Could you check a few things on this model? Use its own coordinates, in mm. A direction names the side the tool comes from. Round coordinates to 2 decimals unless told otherwise and drop trailing zeros. Loops run counter-clockwise (first coordinate to the right, second up) from the corner with the lowest first, then second, coordinate; pieces in that order, holes last. Notation, with made-up numbers: M -37.75,88 L 3.25,88 A24 ccw 3.25,114 Z; hole C 19.5,-32.75 d5. An arc over 180 degrees is marked long. One line per item, written item: value. Start each with the question number.
Q1. Imagine slicing it at D-D (y = 6.25). Please give me the cut outline in (x, z), then the cut area to 3 significant figures.
Q2. Imagine slicing it at B-B (z = 28). Please give me the cut outline in (x, y).
Q3. Which directions (+Z, -Z, +X, -X, +Y, -Y) give clear straight access to the entire face, cutting with the end or side of a thin tool? Please do faces 1 (the face through (12, 7, 19)), 2 (the face through (5, 0.5, 40)), 3 (the face through (14.5, 8, 40)).
Q4. Imagine slicing it at C-C (x = -4.5). Please give me the cut outline in (y, z), then the cut area to 3 significant figures.
Q5. Imagine slicing it at A-A (y = 9). Please give me the cut outline in (x, z), then the cut area to 3 significant figures.
Q6. I'm going to push flat-ended pins straight in: pin 1 Ø6 at (x, y) = (10.5, 4.5) entering from +Z; pin 2 Ø0.6 at (x, z) = (13, 40) entering from +Y; pin 3 Ø6 at (x, y) = (-9.5, 5.5) entering from -Z; pin 4 Ø12 at (x, z) = (4, 30) entering from +Y. Where does each tip first touch, or does it pass through?
Q7. Thinking about a two-plate mould opening in X: for faces 4 (the face through (-15, 5, 20)), 5 (the face through (0, 3, 19)), 6 (the face through (12, 0.5, 40)), which applies, released by +X, released by -X, zero draft, split by the parting line, or undercut?
Q8. Please list where these lines run through material, in increasing order: line 1 along X through (y, z) = (4.75, 29); line 2 along Y through (x, z) = (-9.5, 6.5); line 3 along Z through (x, y) = (-8.25, 1.25).
from build123d import *

# Parameters (mm, degrees)
F1_DEPTH = 39
F2_W     = 0.5
F2_H     = 3
F2_W_2   = 5
F2_H_2   = 0.5
F2_W_3   = 3
F3_DEPTH = 2


with BuildPart() as f1:
    # F0 (on Top) → F1 (new body)
    with BuildSketch(Plane.XY):
        Polygon((-15, 0), (0, 0), (15, 0), (15, 10), (12, 10), (12, 3), (-12, 3), (-12, 10), (-15, 10), align=None)
    extrude(amount=F1_DEPTH)

    # F2 (on face) → F3 (join)
    with BuildSketch(Plane.XY.offset(39)):
        with Locations((-14.75, 8.5)):
            Rectangle(F2_W, F2_H)
        with Locations((-12.5, 0.25)):
            Rectangle(F2_W_2, F2_H_2)
        with Locations((-5.117418, 0.25)):
            Rectangle(F2_W_3, F2_H_2)
        Polygon((-1.844762, 0.5), (-1.844762, 0), (0, 0), (1.844762, 0), (1.844762, 0.5), (0, 0.5), align=None)
        with Locations((5.117418, 0.25)):
            Rectangle(F2_W_3, F2_H_2)
        with Locations((12.5, 0.25)):
            Rectangle(F2_W_2, F2_H_2)
        with Locations((14.75, 8.5)):
            Rectangle(F2_W, F2_H)
    extrude(amount=F3_DEPTH)


solid = f1.part
Report:
1. outline: M -15,0 L -12,0 L -12,39 L -15,39 Z; M 12,0 L 15,0 L 15,39 L 12,39 Z
1. area: 234 mm²
2. outline: M -15,0 L 15,0 L 15,10 L 12,10 L 12,3 L -12,3 L -12,10 L -15,10 Z
3. face 1: +Z, -Z, +Y
3. face 2: +Z, +X, -X, +Y
3. face 3: +Z, +Y
4. outline: M 0,0 L 3,0 L 3,39 L 0.5,39 L 0.5,41 L 0,41 Z
4. area: 118 mm²
5. outline: M -15,0 L -12,0 L -12,39 L -14.5,39 L -14.5,41 L -15,41 Z; M 12,0 L 15,0 L 15,41 L 14.5,41 L 14.5,39 L 12,39 Z
5. area: 236 mm²
6. pin 1: stops at z = 39
6. pin 2: stops at y = 0.5
6. pin 3: stops at z = 0
6. pin 4: stops at y = 3
7. face 4: released by -X
7. face 5: undercut
7. face 6: zero draft
8. line 1: x = -15 to -12, 12 to 15
8. line 2: y = 0 to 3
8. line 3: z = 0 to 39
